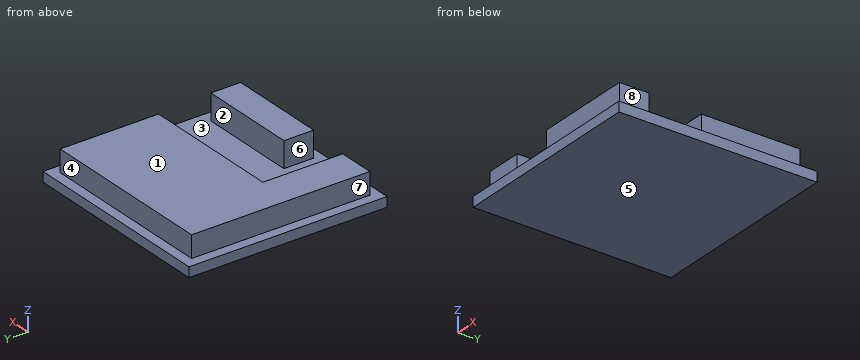
from build123d import *

# Parameters (mm, degrees)
F0_W     = 10
F0_H     = 10
F1_DEPTH = 0.5
F3_DEPTH = 1.1
F4_W     = 5
F4_H     = 1.5
F5_DEPTH = 1.3


with BuildPart() as f1:
    # F0 (on Top) → F1 (new body)
    with BuildSketch(Plane.XY):
        with Locations((5, 5)):
            Rectangle(F0_W, F0_H)
    extrude(amount=F1_DEPTH)

    # F2 (on face) → F3 (join)
    with BuildSketch(Plane.XY.offset(0.5)):
        Polygon((0.5, 9.5), (0.5, 0.5), (2.351106, 0.5), (2.351106, 4.532744), (9.5, 4.532744), (9.5, 9.5), align=None)
    extrude(amount=F3_DEPTH)

    # F4 (on face) → F5 (join)
    with BuildSketch(Plane.XY.offset(0.5)):
        with Locations((6.876147, 1.229358)):
            Rectangle(F4_W, F4_H)
    extrude(amount=F5_DEPTH)


solid = f1.part
Can you work these out from the model? Positions are in its coordinate system, mm. Face numbers are marked on the shaded views. A direction names the side the tool comes from. Coordinates: 2 decimals unless noted, no trailing zeros. Write each loop counter-clockwise with the first axis right and the second up, starting at its lowest first coordinate (ties: lowest second). Pieces come first, ordered by that corner, then holes. Notation, with made-up numbers: (-2.5, -17) -> (47.5, -17) arc R24 ccw to (47.5, 6) -> close; hole circle Ø2 at (86, -30). An arc over 180 degrees is marked (long way). Write each question's results on one line, items separated by ' | '. Start each with the question number.
Q1. Imagine slicing it at A-A (z = 0.75). Write out the boundary of the cut face in (x, y), then the cut area to 3 significant figures.
Q2. Imagine slicing it at D-D (x = 4.5). Write out the boundary of the cut face in (y, z), then the cut area to 3 significant figures.
Q3. Imagine slicing it at C-C (y = 5.5). Write out the boundary of the cut face in (x, z).
Q4. On a 3-axis mill with a long thin cutter (end or side, diameter ignored), from which of +Z, -Z, +X, -X, +Y, -Y can I reach the whole of each face in a straight line? I mean the marked faces 5, 6, 7 and 8. Say none if no direction works.
Q5. If I drill on probe 1 along Y at (x, z) = (4.5, 1.35); probe 2 along X at (y, z) = (1.25, 1.2); probe 3 along Z at (x, y) = (9.5, 3.25), over which ranges is the centre line in solid material (lowest first)?
Q6. Imagine slicing it at B-B (x = 3). Write out the boundary of the cut face in (y, z).
Q7. We'd pull the mould along Y, two halves only. Please class the marked faces 1, 2, 3 and 4: +Y half, -Y half, draft (parallel to the pull), parting line (faces both ways), or undercut.
Q8. I'm going to push flat-ended pins straight in: pin 1 (0.9 mm diameter, centred on x = 6, z = 1, fed in from -Y); pin 2 (2.5 mm diameter, centred on x = 4.5, y = 3.5, fed in from +Z); pin 3 (0.9 mm diameter, centred on y = 6.5, z = 1, fed in from +X). Where does each tip first touch, or does it pass through?
Taken from the geometry:
1) outline: (0.5, 0.5) -> (2.35, 0.5) -> (2.35, 4.53) -> (9.5, 4.53) -> (9.5, 9.5) -> (0.5, 9.5) -> close; (4.38, 0.48) -> (9.38, 0.48) -> (9.38, 1.98) -> (4.38, 1.98) -> close | area: 59.7 mm^2
2) outline: (0, 0) -> (10, 0) -> (10, 0.5) -> (9.5, 0.5) -> (9.5, 1.6) -> (4.53, 1.6) -> (4.53, 0.5) -> (1.98, 0.5) -> (1.98, 1.8) -> (0.48, 1.8) -> (0.48, 0.5) -> (0, 0.5) -> close | area: 12.4 mm^2
3) outline: (0, 0) -> (10, 0) -> (10, 0.5) -> (9.5, 0.5) -> (9.5, 1.6) -> (0.5, 1.6) -> (0.5, 0.5) -> (0, 0.5) -> close
4) face 5: -Z, +X, -X, +Y, -Y | face 6: +Z, -Y | face 7: +Z, -X, +Y, -Y | face 8: +Z, +X, -Y
5) probe 1: y = 0.48 to 1.98, 4.53 to 9.5 | probe 2: x = 0.5 to 2.35, 4.38 to 9.38 | probe 3: z = 0 to 0.5
6) outline: (0, 0) -> (10, 0) -> (10, 0.5) -> (9.5, 0.5) -> (9.5, 1.6) -> (4.53, 1.6) -> (4.53, 0.5) -> (0, 0.5) -> close
7) face 1: draft | face 2: undercut | face 3: undercut | face 4: +Y half
8) pin 1: stops at y = 0.48 | pin 2: stops at z = 1.6 | pin 3: stops at x = 9.5
